Geometry: final body of the model. Coordinates: model frame, mm. A direction names the side the tool comes from. Coordinates: 2 decimals unless noted, no trailing zeros. Loops run counter-clockwise (first coordinate to the right, second up) from the corner with the lowest first, then second, coordinate; pieces in that order, holes last. Notation, with made-up numbers: (69.25, 3.5) -> (123.25, 3.5) arc R29 ccw to (123.25, 31.5) -> close; hole circle Ø9 at (40, 32). An arc over 180 degrees is marked (long way). One line per item, written item: value. Start each with the question number.
Item 1: Ray query, probe 1 along Y at (x, z) = (0, -6.65); probe 2 along X at (y, z) = (0, -4.8); probe 3 along X at (y, z) = (-20, -6.35). Return the intervals inside material, ascending. Write a range as from..to.
Item 2: Section query A-A on x = 0. Return loops of the section in (y, z), then the cut area to 3 significant figures.
Item 3: Mould query, pull axis Y, two halves, no side actions, for faces 1 (the cylindrical face through (0.65, -18.43, -5.54)), 2 (the flat face through (0, -22.66, -6)), 3 (the flat face through (4, 20, -6)). Classes: +Y half, -Y half, draft (parallel to the pull), parting line (faces both ways), or undercut.
Item 4: Section query C-C on z = -6.65. Return loops of the section in (x, y), then the cut area to 3 significant figures.
Item 5: Set-up query: faces 4 (the flat face through (-4, 20, -6)), 5 (the flat face through (-4, -20, -6)), 6 (the flat face through (10, -7, -8)), 7 (the cylindrical face through (-17, 0, -6)), 8 (the flat face through (4, -20, -6)). Return all of +Z, -Z, +X, -X, +Y, -Y with unobstructed straight access to the full face (end or side cutting, diameter ignored); none if empty.
Item 6: Contact query for flat-ended pins moving along their axis: pin 1 Ø1 at (x, z) = (6.5, -6) entering from +Y; pin 2 Ø3 at (x, z) = (8.5, -4) entering from -Y; pin 3 Ø6 at (x, y) = (-1.5, -8.5) entering from +Z; pin 4 Ø3 at (x, z) = (11, -4.5) entering from -Y. Output: stop coordinate, or through.
Item 7: Section query D-D on x = 7. Return loops of the section in (y, z), then the cut area to 3 significant figures.
Item 8: Section query B-B on y = 0. Return loops of the section in (x, z).
from build123d import *

# Parameters (mm, degrees)
CYLINDER_R          = 2
CYLINDER_DEPTH      = 10
CYLINDER098_R       = 1.7
CYLINDER098_DEPTH   = 14
CYLINDER097_R       = 12
CYLINDER097_DEPTH   = 33
CYLINDER099_R       = 1.7
CYLINDER099_DEPTH   = 14
BOX017_W            = 45.5
BOX017_H            = 8
BOX017_DEPTH        = 5
CYLINDER096_R       = 17
CYLINDER096_DEPTH   = 5
CUT_PLACEMENT_ANGLE = 90


with BuildPart() as cylinder:
    # Cylinder → Cylinder (new body)
    with BuildSketch(Plane(origin=(0, 57, 0), x_dir=(1, 0, 0), z_dir=(0, 0, 1))):
        Circle(CYLINDER_R)
    extrude(amount=CYLINDER_DEPTH)


with BuildPart() as obj1:
    # Cylinder098 → Cylinder098 (new body)
    with BuildSketch(Plane(origin=(53.66, 148, -15), x_dir=(1, 0, 0), z_dir=(0, 0, 1))):
        Circle(CYLINDER098_R)
    extrude(amount=CYLINDER098_DEPTH)


with BuildPart() as obj2:
    # Cylinder097 → Cylinder097 (new body)
    with BuildSketch(Plane(origin=(73.66, 148, -10), x_dir=(1, 0, 0), z_dir=(0, 0, 1))):
        Circle(CYLINDER097_R)
    extrude(amount=CYLINDER097_DEPTH)


with BuildPart() as fusion041:
    # Cylinder099 → Cylinder099 (new body)
    with BuildSketch(Plane(origin=(93.66, 148, -14), x_dir=(1, 0, 0), z_dir=(0, 0, 1))):
        Circle(CYLINDER099_R)
    extrude(amount=CYLINDER099_DEPTH)

    # Fusion041: union obj1, obj2
    add(obj1.part)
    add(obj2.part)


with BuildPart() as obj3:
    # Box017 → Box017 (new body)
    with BuildSketch(Plane(origin=(51, 144, -10), x_dir=(1, 0, 0), z_dir=(0, 0, 1))):
        with Locations((22.75, 4)):
            Rectangle(BOX017_W, BOX017_H)
    extrude(amount=BOX017_DEPTH)


with BuildPart() as cut:
    # Cylinder096 → Cylinder096 (new body)
    with BuildSketch(Plane(origin=(73.66, 148, -10), x_dir=(1, 0, 0), z_dir=(0, 0, 1))):
        Circle(CYLINDER096_R)
    extrude(amount=CYLINDER096_DEPTH)

    # Fusion042: union obj3
    add(obj3.part)

    # Cut011: cut Fusion041
    add(fusion041.part, mode=Mode.SUBTRACT)


with BuildPart() as cut_1:
    # Cut011 placement: moved
    add(cut.part.moved(Location((-73.66, -148, 2))))

    # Cut: cut Cylinder
    add(cylinder.part, mode=Mode.SUBTRACT)


with BuildPart() as cut_2:
    # Cut placement: moved
    add(cut_1.part.rotate(Axis((0, 0, 0), (0, 0, 1)), CUT_PLACEMENT_ANGLE))


solid = cut_2.part
Reply:
1. probe 1: y = -22.66..-21.7, -18.3..-12, 12..18.3, 21.7..22.84
1. probe 2: x = -17..-12, 12..17
1. probe 3: x = -4..-1.7, 1.7..4
2. outline: (-22.66, -8) -> (-21.7, -8) -> (-21.7, -3) -> (-22.66, -3) -> close; (-18.3, -8) -> (-12, -8) -> (-12, -3) -> (-18.3, -3) -> close; (12, -8) -> (18.3, -8) -> (18.3, -3) -> (12, -3) -> close; (21.7, -8) -> (22.84, -8) -> (22.84, -3) -> (21.7, -3) -> close
2. area: 73.5 mm²
3. face 1: undercut
3. face 2: -Y half
3. face 3: draft
4. outline: (-4, -22.66) -> (4, -22.66) -> (4, -16.52) arc R17 ccw to (4, 16.52) -> (4, 22.84) -> (-4, 22.84) -> (-4, 16.52) arc R17 ccw to (-4, -16.52) -> close; hole circle Ø24 at (0, 0); hole circle Ø3.4 at (0, -20); hole circle Ø3.4 at (0, 20)
4. area: 532 mm²
5. face 4: +Z, -Z, -X, +Y
5. face 5: +Z, -Z, -X, -Y
5. face 6: -Z, +X, -X, +Y, -Y
5. face 7: +Z, -Z, -X
5. face 8: +Z, -Z, +X, -Y
6. pin 1: stops at y = 15.91
6. pin 2: stops at y = -15.49
6. pin 3: passes through
6. pin 4: stops at y = -14.1
7. outline: (-15.49, -8) -> (-9.75, -8) -> (-9.75, -3) -> (-15.49, -3) -> close; (9.75, -8) -> (15.49, -8) -> (15.49, -3) -> (9.75, -3) -> close
7. area: 57.5 mm²
8. outline: (-17, -8) -> (-12, -8) -> (-12, -3) -> (-17, -3) -> close; (12, -8) -> (17, -8) -> (17, -3) -> (12, -3) -> close
